from build123d import *
from OCP.BRepFilletAPI import BRepFilletAPI_MakeChamfer

# Parameters (mm, degrees)
CHAMFER1_SIZE      = 8
CHAMFER1_SIZE2     = 2
CHAMFER2_SIZE      = 0.3
CHAMFER2_SIZE2     = 0.412310563
CUT_EXTRUDE1_DEPTH = 2.92
CIRPATTERN1_COUNT  = 6


with BuildPart() as part:
    # Sketch1 → Revolve1 (revolve)
    with BuildSketch(Plane.XY, mode=Mode.PRIVATE) as revolve1_sk:
        Polygon((19.7, -15), (19.7, -26.6), (21, -26.6), (21, -29.6), (20.5, -29.6), (13.5, -36.6), (13.5, -37.6), (25, -37.6), (25, -15), align=None)
    revolve(revolve1_sk.sketch.rotate(Axis((0, 0, 0), (0, -1, 0)), 90), axis=Axis((0, 0, 0), (0, -1, 0)))

    # Chamfer1
    chamfer1_edges = [part.edges().sort_by_distance(p)[0] for p in [
        (0, -37.6, -25),
    ]]
    chamfer1_side = [part.faces().sort_by_distance(p)[0] for p in [
        (0, -37.6, -14.207106781),
    ]]
    chamfer(chamfer1_edges, length=CHAMFER1_SIZE, length2=CHAMFER1_SIZE2, reference=chamfer1_side[0])

    # Chamfer2: one chamfer whose edges measure the first distance from different faces: ONE call of the kernel's chamfer builder (chamfer() names one face for all edges)
    chamfer2_edges_1 = [part.edges().sort_by_distance(p)[0] for p in [
        (0, -35.6, -25),
    ]]
    chamfer2_side_1 = [part.faces().sort_by_distance(p)[0] for p in [
        (0, -36.6, -21),
    ]]
    chamfer2_edges_2 = [part.edges().sort_by_distance(p)[0] for p in [
        (0, -37.6, -13.5),
        (0, -15, -25),
        (0, -15, -19.7),
    ]]
    chamfer2 = BRepFilletAPI_MakeChamfer(part.part.solid().wrapped)
    for e in chamfer2_edges_1:
        chamfer2.Add(CHAMFER2_SIZE, CHAMFER2_SIZE2, e.wrapped, chamfer2_side_1[0].wrapped)  # the first distance lies on this face
    for e in chamfer2_edges_2:
        chamfer2.Add(CHAMFER2_SIZE, e.wrapped)
    add(Compound.cast(chamfer2.Shape()), mode=Mode.REPLACE)

    # Sketch4 → Cut-Extrude1 (cut)
    with BuildSketch(Plane.ZY.offset(25)):
        with BuildLine():
            Line((-2.58, -37.6), (-2.58, -25.98))
            ThreePointArc((-2.58, -25.98), (0, -23.4), (2.58, -25.98))
            Line((2.58, -25.98), (2.58, -37.6))
            ThreePointArc((2.58, -37.6), (0, -40.18), (-2.58, -37.6))
        make_face()
    cut_extrude1 = extrude(amount=-CUT_EXTRUDE1_DEPTH, mode=Mode.SUBTRACT)

    # CirPattern1: Cut-Extrude1 ×6 about axis
    cirpattern1_axis = Axis((0, 0, 0), (0, 1, 0))
    for i in range(1, CIRPATTERN1_COUNT):
        add(cut_extrude1.rotate(cirpattern1_axis, i * 360 / CIRPATTERN1_COUNT), mode=Mode.SUBTRACT)


solid = part.part
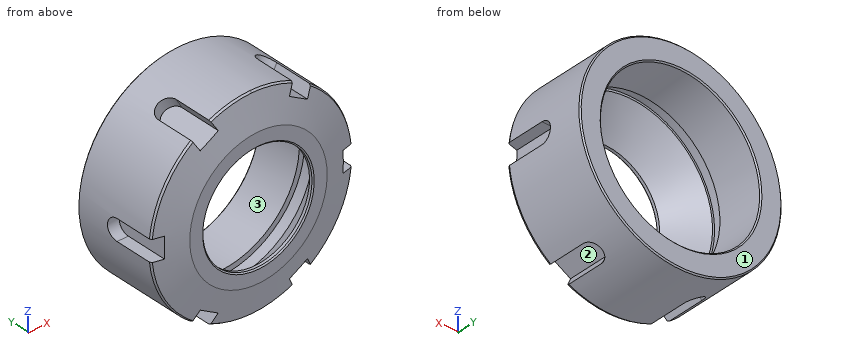
Geometry check sheet. Reference: the model listing, model coordinates, mm. Face numbers are marked on the shaded views. A direction names the side the tool comes from. Give positions to 0.01 mm unless a question says otherwise; leave off trailing zeros. Order: outer loops, then holes, each group sorted by start corner. A loop starts at its lowest first (then second) coordinate and runs counter-clockwise, first axis right, second up. Notation, with made-up numbers: (38, 45.25) - (60, 45.25) arc R19 ccw to (60, 68.25) - close; hole circle Ø3 at (-21, 25). An arc over 180 degrees is marked (long way). Use one line per item in the form item = value.
1) Sectioned sample at B-B (y = -33.75). Record the boundary of the cut face in (x, z), and give its area (3 significant figures).
Working result:
outline = (-24.87, -2.58) arc R25 ccw to (-14.67, -20.25) - (-13.27, -17.83) - (-8.81, -20.41) - (-10.2, -22.83) arc R25 ccw to (10.2, -22.83) - (8.81, -20.41) - (13.27, -17.83) - (14.67, -20.25) arc R25 ccw to (24.87, -2.58) - (22.08, -2.58) - (22.08, 2.58) - (24.87, 2.58) arc R25 ccw to (14.67, 20.25) - (13.27, 17.83) - (8.81, 20.41) - (10.2, 22.83) arc R25 ccw to (-10.2, 22.83) - (-8.81, 20.41) - (-13.27, 17.83) - (-14.67, 20.25) arc R25 ccw to (-24.87, 2.58) - (-22.08, 2.58) - (-22.08, -2.58) - close; hole circle Ø32.7 at (0, 0)
area = 1,030 mm^2
2) Sectioned sample at C-C (y = -24.25). Record the boundary of the cut face in (x, z), and give its area (3 significant figures).
Working result:
outline = (-24.93, -1.91) arc R25 ccw to (-14.12, -20.63) - (-12.7, -18.16) - (-9.38, -20.08) - (-10.81, -22.54) arc R25 ccw to (10.81, -22.54) - (9.38, -20.08) - (12.7, -18.16) - (14.12, -20.63) arc R25 ccw to (24.93, -1.91) - (22.08, -1.91) - (22.08, 1.91) - (24.93, 1.91) arc R25 ccw to (14.12, 20.63) - (12.7, 18.16) - (9.38, 20.08) - (10.81, 22.54) arc R25 ccw to (-10.81, 22.54) - (-9.38, 20.08) - (-12.7, 18.16) - (-14.12, 20.63) arc R25 ccw to (-24.93, 1.91) - (-22.08, 1.91) - (-22.08, -1.91) - close; hole circle Ø39.4 at (0, 0)
area = 678 mm^2
3) Sectioned sample at D-D (y = -18). Record the boundary of the cut face in (x, z).
Working result:
outline = circle Ø50 at (0, 0); hole circle Ø39.4 at (0, 0)
4) Depth check by flat-ended pin: pin 1 Ø6 at (x, y) = (6.5, -19.5) entering from -Z; pin 2 Ø2 at (y, z) = (-29.5, -16) entering from +X; pin 3 Ø1 at (x, y) = (-1, -23) entering from -Z (3 decimals); pin 4 Ø12.5 at (x, z) = (5, -4) entering from -Y. Enter the tip coordinate at first touch or a pass-through.
Working result:
pin_1 = -24.75
pin_2 = 20
pin_3 = -24.995
pin_4 = through
5) Access from +Z, -Z, +X, -X, +Y, -Y to the whole of each face (thin tool, end or side, straight path). Record for the marked faces 1, 2 and 3.
Working result:
face_1 = +Z, -Z, +X, -X, +Y
face_2 = -Y
face_3 = +Y
6) Material ranges on probe 1 along X at (y, z) = (-24, 0); probe 2 along Z at (x, y) = (13, -34.5); probe 3 along Z at (x, y) = (11, -20.25), recorded low to high. Write a range as from..to.
Working result:
probe_1 = -22.08..-19.7, 19.7..22.08
probe_2 = -17.99..-8.62, 8.62..17.99
probe_3 = -22.45..-16.34, 16.34..22.45
